Autodesk Inventor part; units mm, degrees
ref_plane "Plano de trabajo2" through (-10.2243, 33.4626, 0) normal (-1, 0, 0) x (0, 0, -1)
ref_plane "YZ Plane" through (0, 0, 0) normal (1, 0, 0) x (0, 1, 0)
ref_plane "XZ Plane" through (0, 0, 0) normal (0, 1, 0) x (-1, 0, 0)
sketch "Boceto3" plane through (0, 0, 0) normal (0, 0, 1) x (1, 0, 0)
  line L0 (-15.1624, 32.0626) -> (-18.8843, 32.0626)
  line L1 (-13.7243, 33.4626) -> (-13.7243, 30.9626)
  line L2 (-13.7243, 30.9626) -> (-14.4343, 30.9626)
  line L3 (-14.4343, 30.9626) -> (-15.1624, 32.0626)
  arc A0 (-18.8843, 32.0626) -> (-21.6243, 29.3226) centre (-18.8843, 29.3226) ccw
  line L4 (-13.7243, 33.4626) -> (-10.2243, 33.4626)
  line L5 (-21.6243, 29.3226) -> (-21.6243, 26.5626)
  arc A1 (-10.2243, 33.4626) -> (-10.2243, 26.5626) centre (5.1794, 30.0126) ccw
  line L6 (-21.6243, 26.5626) -> (-21.1243, 26.5626)
  line L7 (-10.2243, 26.5626) -> (-10.7243, 26.5626)
  arc A2 (-10.7243, 26.5626) -> (-21.1243, 26.5626) centre (-15.9243, 23.1493) ccw
  dimension "d218" = 2.5
  dimension "d219" = 0.71
  dimension "d221" = 33.5
  dimension "d223" = 2.74
  dimension "d281" = 3.5
  dimension "d288" = 2.76
  dimension "d291" = 0.5
  dimension "d292" = 0.5
extrude "Extrusión4" add sketch "Boceto3" against normal blind 1023.4
ref_plane "Plano de trabajo2" through (-10.2243, 33.4626, 0) normal (-1, 0, 0) x (0, 0, -1)
ref_plane "Plano de trabajo4" through (0, 0, -511.7) normal (0, 0, 1) x (1, 0, 0)
sketch "Boceto5" plane through (-10.2243, 33.4626, 0) normal (-1, 0, 0) x (0, 0, -1)
  line L0 (0, 0) -> (0, 6.9)
  line L1 (0, 6.9) -> (6.9, 0)
  line L2 (0, 0) -> (1023.4, 0)
  line L3 (6.9, 0) -> (0, 0)
  line L4 (0, 0) -> (0, 6.9)
  point P0 (0, 33.4626)
  dimension "d296" = 45
extrude "Extrusión6" cut sketch "Boceto5" along normal through all
mirror "Simetría3" about plane through (0, 0, -511.7) normal (0, 0, 1) of "Extrusión6"
properties part number "SP40-10 JUNTA INT CRISTAL 1023" material "Caucho"
The listing builds one solid part. Answer for the finished solid, in the listing's coordinates (mm). Round coordinates to 2 decimals unless told otherwise and drop trailing zeros. Loops run counter-clockwise (first coordinate to the right, second up) from the corner with the lowest first, then second, coordinate; pieces in that order, holes last. Notation, with made-up numbers: M 55,20 L 113,20 A27 cw 113,58 Z; hole C 21,-3 d7. An arc over 180 degrees is marked long. Return JSON: item names as keys, results as strings.
Q1. Find section A-A, the plane y = 27.75. Determine the outline of the cut face in (x, z), plus the area to 3 significant figures.
Results list:
{"outline": "M -21.62,-1022.21 L -20.11,-1022.21 L -20.11,-1.19 L -21.62,-1.19 Z; M -11.74,-1022.21 L -10.44,-1022.21 L -10.44,-1.19 L -11.74,-1.19 Z", "area": "2,870 mm2"}
Q2. Find section B-B, the plane z = -410.5. Determine the outline of the cut face in (x, y), plus the area to 3 significant figures.
Results list:
{"outline": "M -21.62,26.56 L -21.12,26.56 A6.22 cw -10.72,26.56 L -10.22,26.56 A15.79 cw -10.22,33.46 L -13.72,33.46 L -13.72,30.96 L -14.43,30.96 L -15.16,32.06 L -18.88,32.06 A2.74 ccw -21.62,29.32 Z", "area": "42.5 mm2"}
Q3. Each of these flat-tipped pins is pushed along its axis until it touches: pin 1 Ø2 at (y, z) = (31, -141) entering from +X; pin 2 Ø0.8 at (y, z) = (31.5, -570) entering from -X; pin 3 Ø1.5 at (x, z) = (-18, -822.5) entering from -Y. Where does it stop, or does it pass through?
Results list:
{"pin 1": "stops at x = -10.48", "pin 2": "stops at x = -20.97", "pin 3": "stops at y = 28.69"}
Q4. Find the intervals of material crossed by line 1 along Y through (x, z) = (-21, -773.5); line 2 along X through (y, z) = (31, -42); line 3 along Y through (x, z) = (-16.75, -792.5), in increasing order. Write a range as from..to.
Results list:
{"line 1": "y = 26.74..31.06", "line 2": "x = -21.05..-14.46, -13.72..-10.58", "line 3": "y = 29.31..32.06"}
